```python
from build123d import *

# Parameters (mm, degrees)
BASPROSKE_W        = 6
BASPROSKE_H        = 16.5
TOOTHCUT_DEPTH     = 25.093567606
TEETHCUTS_COUNT    = 20
TEETHCUTS_ANGLE    = 342
BORSKE_R           = 3
BORE_DEPTH         = 50.0000508
SKETCH1_R          = 1
CUT_EXTRUDE1_DEPTH = 10
CIRPATTERN1_COUNT  = 3


with BuildPart() as part:
    # BasProSke → Base-Revolve (revolve)
    with BuildSketch(Plane(origin=(0, 0, 0), x_dir=(1, 0, 0), z_dir=(0, 1, 0)), mode=Mode.PRIVATE) as base_revolve_sk:
        with Locations((3, 8.25)):
            Rectangle(BASPROSKE_W, BASPROSKE_H)
    revolve(base_revolve_sk.sketch.rotate(Axis((-10, 0, 0), (1, 0, 0)), 180), axis=Axis((-10, 0, 0), (1, 0, 0)))

    # TooCutSke → ToothCut (cut, through all)
    with BuildSketch(Plane(origin=(0, 0, 0), x_dir=(0, 0, -1), z_dir=(1, 0, 0))):
        with BuildLine():
            ThreePointArc((0.74381438, 13.102904875), (0, 13.124), (-0.74381438, 13.102904875))
            ThreePointArc((-0.74381438, 13.102904875), (-1.226473103, 14.852072512), (-2.209965745, 16.376962373))
            ThreePointArc((-2.209965745, 16.376962373), (0, 16.5254), (2.209965745, 16.376962373))
            ThreePointArc((2.209965745, 16.376962373), (1.226473103, 14.852072512), (0.74381438, 13.102904875))
        make_face()
    toothcut = extrude(amount=TOOTHCUT_DEPTH, mode=Mode.SUBTRACT)

    # TeethCuts: ToothCut ×20 about axis
    teethcuts_axis = Axis((-10, 0, 0), (1, 0, 0))
    for i in range(1, TEETHCUTS_COUNT):
        add(toothcut.rotate(teethcuts_axis, i * TEETHCUTS_ANGLE / (TEETHCUTS_COUNT - 1)), mode=Mode.SUBTRACT)

    # BorSke → Bore (cut, symmetric)
    with BuildSketch(Plane(origin=(0, 0, 0), x_dir=(0, 0, -1), z_dir=(1, 0, 0))):
        with Locations(Location((0, 0, 0), (0, 0, 180))):
            Circle(BORSKE_R)
    extrude(amount=BORE_DEPTH, both=True, mode=Mode.SUBTRACT)

    # Sketch1 → Cut-Extrude1 (cut)
    with BuildSketch(Plane(origin=(6, 0, 0), x_dir=(0, 0, -1), z_dir=(1, 0, 0))):
        with BuildLine():
            ThreePointArc((6, 6.708203932), (3.211398808, 8.407551231), (0, 9))
            ThreePointArc((0, 9), (-3.211398808, 8.407551231), (-6, 6.708203932))
            ThreePointArc((-6, 6.708203932), (-4.925085043, 6.875718869), (-4.333333333, 5.96284794))
            ThreePointArc((-4.333333333, 5.96284794), (-4.420462404, 5.55459965), (-4.666666667, 5.217491947))
            ThreePointArc((-4.666666667, 5.217491947), (-2.497754628, 6.539206513), (0, 7))
            ThreePointArc((0, 7), (2.497754628, 6.539206513), (4.666666667, 5.217491947))
            ThreePointArc((4.666666667, 5.217491947), (4.587977341, 6.629514607), (6, 6.708203932))
        make_face()
        with Locations((-5.333333333, 5.96284794)):
            Circle(SKETCH1_R)
        with Locations((5.333333333, 5.96284794)):
            Circle(SKETCH1_R)
    cut_extrude1 = extrude(amount=-CUT_EXTRUDE1_DEPTH, mode=Mode.SUBTRACT)

    # CirPattern1: Cut-Extrude1 ×3 about axis
    cirpattern1_axis = Axis((0, 0, 0), (1, 0, 0))
    for i in range(1, CIRPATTERN1_COUNT):
        add(cut_extrude1.rotate(cirpattern1_axis, i * 360 / CIRPATTERN1_COUNT), mode=Mode.SUBTRACT)


solid = part.part
```
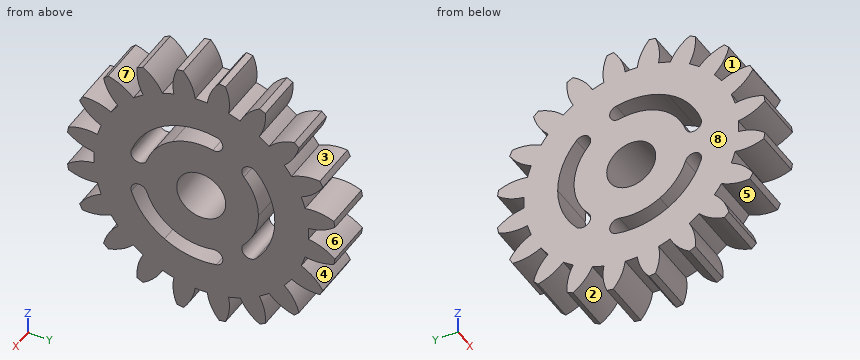
Could you check a few things on this model? Use its own coordinates, in mm. Face numbers are marked on the shaded views. A direction names the side the tool comes from. Coordinates: 2 decimals unless noted, no trailing zeros. Loops run counter-clockwise (first coordinate to the right, second up) from the corner with the lowest first, then second, coordinate; pieces in that order, holes last.
1) Imagine slicing it at B-B (z = 14). List the corners of the cut face in (x, y) for me.
Reported:
outline: (0, -7.87) - (6, -7.87) - (6, -6) - (0, -6) - close; (0, -3.46) - (6, -3.46) - (6, -0.92) - (0, -0.92) - close; (0, 0.92) - (6, 0.92) - (6, 3.46) - (0, 3.46) - close; (0, 6) - (6, 6) - (6, 7.87) - (0, 7.87) - close
2) Please list where these lines run through material, in increasing order: line 1 along Y through (x, z) = (1.4, 2.5); line 2 along Z through (x, y) = (4.75, -2); line 3 along Z through (x, y) = (3.35, -11.5).
Reported:
line 1: y = -16.31 to -8.6, -6.54 to -1.66, 1.66 to 6.54, 8.65 to 16.31
line 2: z = -16.13 to -8.77, -6.71 to -2.24, 2.24 to 6.71, 8.77 to 16.13
line 3: z = -11.83 to -10.11, -7.33 to 7.33, 10.11 to 11.83
3) Thinking about a two-plate mould opening in Y: for the marked faces 5, 6, 7 and 8, which applies, released by +Y, released by -Y, zero draft, split by the parting line, or undercut?
Reported:
face 5: undercut
face 6: released by +Y
face 7: undercut
face 8: zero draft
4) Imagine slicing it at A-A (y = 0). List the corners of the cut face in (x, z) for me, and give its area (3 significant figures).
Reported:
outline: (0, -13.12) - (6, -13.12) - (6, -9) - (0, -9) - close; (0, -7) - (6, -7) - (6, -3) - (0, -3) - close; (0, 3) - (6, 3) - (6, 7) - (0, 7) - close; (0, 9) - (6, 9) - (6, 13.12) - (0, 13.12) - close
area: 97.5 mm2
5) Which directions (+Z, -Z, +X, -X, +Y, -Y) give clear straight access to the entire face, cutting with the end or side of a thin tool? Please do the marked faces 1, 2, 3 and 4.
Reported:
face 1: +X, -X, -Y
face 2: -Z, +X, -X
face 3: +X, -X
face 4: +X, -X, +Y
6) Will these pins go through, and if not, where does the flat tip stop? pin 1 Ø2 at (x, z) = (5, 3.5) entering from +Y; pin 2 Ø3.5 at (y, z) = (0, 0) entering from -X; pin 3 Ø3 at (x, y) = (5, -12) entering from +Z.
Reported:
pin 1: stops at y = 16.31
pin 2: passes through
pin 3: stops at z = 11.94
7) Imagine slicing it at C-C (x = 0.65). State how many separate pieces and enclosed holes the cut face has, and give its area (3 significant figures).
Reported:
separate pieces: 1
enclosed holes: 4
area: 574 mm2
